Read the model definition and answer for the solid it produces. Units are mm, in the model's axes. Face numbers are marked on the shaded views. A direction names the side the tool comes from. Round coordinates to 2 decimals unless told otherwise and drop trailing zeros. Loops run counter-clockwise (first coordinate to the right, second up) from the corner with the lowest first, then second, coordinate; pieces in that order, holes last. Notation, with made-up numbers: M 74.25,-12.5 L 104.25,-12.5 A37 cw 104.25,26.5 Z; hole C 6.5,48 d1. An arc over 180 degrees is marked long. Answer as CSV lines item,"result".
```python
from build123d import *

# Parameters (mm, degrees)
SKETCH1_R           = 5
BOSS_EXTRUDE1_DEPTH = 40
SKETCH2_R           = 3
BOSS_EXTRUDE2_DEPTH = 5
SKETCH3_R           = 1.5
BOSS_EXTRUDE3_DEPTH = 20
CHAMFER1_SIZE       = 1
SKETCH4_R           = 2
BOSS_EXTRUDE4_DEPTH = 5
BOSS_EXTRUDE5_START = 4
SKETCH5_R           = 5
BOSS_EXTRUDE5_DEPTH = 4
CHAMFER2_SIZE       = 3
CHAMFER3_SIZE       = 1


with BuildPart() as part:
    # Sketch1 → Boss-Extrude1 (new body)
    with BuildSketch(Plane(origin=(0, 0, 0), x_dir=(1, 0, 0), z_dir=(0, 1, 0))):
        with Locations(Location((0, 0, 0), (0, 0, 270))):
            Circle(SKETCH1_R)
    extrude(amount=BOSS_EXTRUDE1_DEPTH)

    # Sketch2 → Boss-Extrude2 (add)
    with BuildSketch(Plane(origin=(0, 40, 0), x_dir=(1, 0, 0), z_dir=(0, 1, 0))):
        with Locations(Location((0, 0, 0), (0, 0, 270))):
            Circle(SKETCH2_R)
    extrude(amount=BOSS_EXTRUDE2_DEPTH)

    # Sketch3 → Boss-Extrude3 (add)
    with BuildSketch(Plane(origin=(0, 45, 0), x_dir=(1, 0, 0), z_dir=(0, 1, 0))):
        with Locations(Location((0, 0, 0), (0, 0, 270))):
            Circle(SKETCH3_R)
    extrude(amount=BOSS_EXTRUDE3_DEPTH)

    # Chamfer1
    chamfer1_edges = [part.edges().sort_by_distance(p)[0] for p in [
        (0, 65, -1.5),
    ]]
    chamfer(chamfer1_edges, length=CHAMFER1_SIZE)

    # Sketch4 → Boss-Extrude4 (add)
    with BuildSketch(Plane.XZ):
        with Locations(Location((0, 0, 0), (0, 0, 270))):
            Circle(SKETCH4_R)
    extrude(amount=BOSS_EXTRUDE4_DEPTH)

    # Sketch5 → Boss-Extrude5 (add)
    with BuildSketch(Plane.XZ.offset(5).offset(BOSS_EXTRUDE5_START)):
        with Locations(Location((0, 0, 0), (0, 0, 90))):
            Circle(SKETCH5_R)
    extrude(amount=-BOSS_EXTRUDE5_DEPTH)

    # Chamfer2
    chamfer2_edges = [part.edges().sort_by_distance(p)[0] for p in [
        (0, 0, -5),
    ]]
    chamfer(chamfer2_edges, length=CHAMFER2_SIZE - 0.0001)  # a hair under: the kernel refuses the full size

    # Chamfer3
    chamfer3_edges = [part.edges().sort_by_distance(p)[0] for p in [
        (0, -5, -5),
    ]]
    chamfer(chamfer3_edges, length=CHAMFER3_SIZE)


solid = part.part
```
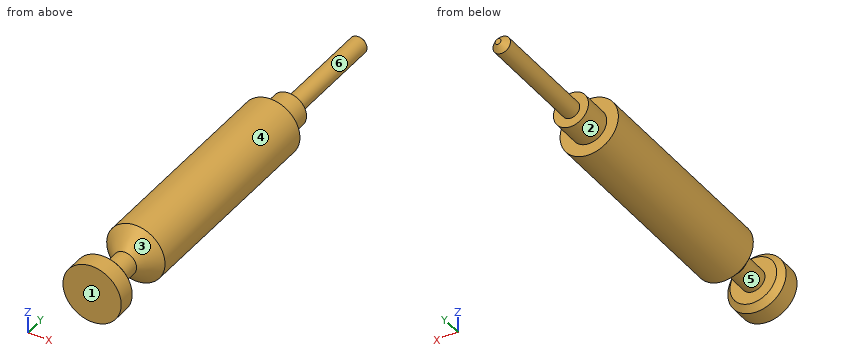
1) Straight lines are drawn through the part: line 1 (X direction, y = -1, z = 0); line 2 (Y direction, x = 1, z = -2.5); line 3 (Y direction, x = 3, z = -2). For each, find the intervals that lie inside material, in ascending order.
Evaluation:
line 1,"x = -2 to 2"
line 2,"y = -9 to -5, 0.69 to 45"
line 3,"y = -9 to -5, 1.61 to 40"
2) Find section A-A, the plane y = 26. Give the vertices of the cut face in (x, z), then the cut area to 3 significant figures.
Evaluation:
outline,"C 0,0 d10"
area,"78.5 mm^2"
3) A tool of negligible diameter and unlimited length cuts with its end or side. For the marked faces 4, 5 and 6, from which of +Z, -Z, +X, -X, +Y, -Y can it reach the whole face along a straight path? Write none if from no direction.
Evaluation:
face 4,"+Y, -Y"
face 5,"none"
face 6,"+Y"
4) Each of these flat-tipped pins is pushed along its axis until it touches: P1, Ø3, axis at x = -2, z = -2, coming from the +Y side; P2, Ø3, axis at x = -4, z = 3, coming from the +Y side; P3, Ø3, axis at x = -3, z = 2.5, coming from the +Y side. Where does it stop, or does it pass through?
Evaluation:
P1,"stops at y = 64.17"
P2,"stops at y = 40"
P3,"stops at y = 45"
5) Determine the mould class of the marked faces 1, 2 and 3 for opening direction Y: released by +Y, released by -Y, zero draft, split by the parting line, or undercut.
Evaluation:
face 1,"released by -Y"
face 2,"zero draft"
face 3,"undercut"
